from build123d import *

# Parameters (mm, degrees)
SKETCH1_W           = 25
SKETCH1_H           = 2
SKETCH2_W           = 15
SKETCH2_H           = 3.5
TAPPED_HOLE1_REACH  = 31.385
TAPPED_HOLE1_BORE_R = 1.25
CIRPATTERN1_COUNT   = 2
CIRPATTERN1_ANGLE   = 90
CHAMFER1_SIZE       = 1


with BuildPart() as part:
    # Sketch1 → Revolve1 (revolve)
    with BuildSketch(Plane.XY, mode=Mode.PRIVATE) as revolve1_sk:
        with Locations((12.5, 5)):
            Rectangle(SKETCH1_W, SKETCH1_H)
    revolve(revolve1_sk.sketch.rotate(Axis((0, 0, 0), (1, 0, 0)), 90), axis=Axis((0, 0, 0), (1, 0, 0)))

    # Sketch2 → Revolve2 (revolve)
    with BuildSketch(Plane.XY, mode=Mode.PRIVATE) as revolve2_sk:
        with Locations((7.5, 5.75)):
            Rectangle(SKETCH2_W, SKETCH2_H)
    revolve(revolve2_sk.sketch.rotate(Axis((0, 0, 0), (1, 0, 0)), 90), axis=Axis((0, 0, 0), (1, 0, 0)))

    # Tapped Hole1 bore → Tapped Hole1 (cut, up to next)
    with BuildSketch(Plane(origin=(0, 6, 0), x_dir=(1, 0, 0), z_dir=(0, 1, 0)), mode=Mode.PRIVATE) as tapped_hole1_sk1:
        with Locations((20, 0)):
            Circle(TAPPED_HOLE1_BORE_R)
    tapped_hole1_tool1 = extrude(tapped_hole1_sk1.sketch, amount=-TAPPED_HOLE1_REACH, mode=Mode.PRIVATE) & part.part
    tapped_hole1 = tapped_hole1_tool1.solids().sort_by_distance((20, 6, 0))[0]
    add(tapped_hole1, mode=Mode.SUBTRACT)

    # CirPattern1: Tapped Hole1 ×2 about axis
    cirpattern1_axis = Axis((0, 0, 0), (-1, 0, 0))
    for i in range(1, CIRPATTERN1_COUNT):
        add(tapped_hole1.rotate(cirpattern1_axis, i * CIRPATTERN1_ANGLE / (CIRPATTERN1_COUNT - 1)), mode=Mode.SUBTRACT)

    # Chamfer1
    chamfer1_edges = [part.edges().sort_by_distance(p)[0] for p in [
        (25, 0, -6),
    ]]
    chamfer(chamfer1_edges, length=CHAMFER1_SIZE)


solid = part.part
Geometry check sheet. Reference: the model listing, model coordinates, mm. A direction names the side the tool comes from. Give positions to 0.01 mm unless a question says otherwise; leave off trailing zeros. Order: outer loops, then holes, each group sorted by start corner. A loop starts at its lowest first (then second) coordinate and runs counter-clockwise, first axis right, second up. Notation, with made-up numbers: M 65.25,54.25 L 73.25,54.25 A24 ccw 73.25,83.25 Z; hole C 25.5,40 d8. An arc over 180 degrees is marked long. Use a Markdown table: item, result.
Item 1: Section check A-A (y = 0). Record the cut outline in (x, z).
Answers follow:
| item | result |
|---|---|
| outline | M 0,-7.5 L 15,-7.5 L 15,-6 L 18.75,-6 L 18.75,-4 L 0,-4 Z; M 0,4 L 25,4 L 25,5 L 24,6 L 15,6 L 15,7.5 L 0,7.5 Z; M 21.25,-6 L 24,-6 L 25,-5 L 25,-4 L 21.25,-4 Z |
Item 2: Material ranges on line 1 along Y through (x, z) = (18.5, 0); line 2 along X through (y, z) = (4.3, 0); line 3 along Y through (x, z) = (13.75, 0), recorded low to high.
Answers follow:
| item | result |
|---|---|
| line 1 | y = -6 to -4, 4 to 6 |
| line 2 | x = 0 to 18.75, 21.25 to 25 |
| line 3 | y = -7.5 to -4, 4 to 7.5 |
Item 3: Section check C-C (x = 20). Record the cut outline in (y, z), and give its area (3 significant figures).
Answers follow:
| item | result |
|---|---|
| outline | M -1.25,-5.87 L -1.25,-3.8 A4 cw long 3.8,1.25 L 5.87,1.25 A6 ccw long Z; M 1.25,-5.87 A6 ccw 5.87,-1.25 L 3.8,-1.25 A4 cw 1.25,-3.8 Z |
| area | 52.7 mm2 |
Item 4: Section check D-D (x = 2.5). Record the cut outline in (y, z).
Answers follow:
| item | result |
|---|---|
| outline | C 0,0 d15; hole C 0,0 d8 |
Item 5: Draft check along X on faces 1 (the cylindrical face through (18.75, 4.92, -0.05)), 2 (the cylindrical face through (7.605, -6.324, 4.032)), 3 (the cylindrical face through (18.75, -0.05, -4.92)), 4 (the flat face through (15, -6, -2)). Enter one of: +X half, -X half, draft (parallel to the pull), parting line (faces both ways), or undercut.
Answers follow:
| item | result |
|---|---|
| face 1 | undercut |
| face 2 | draft |
| face 3 | undercut |
| face 4 | +X half |
Item 6: Depth check by flat-ended pin: P1, Ø2, axis at x = 20, z = 0, coming from the +Y side; P2, Ø8, axis at x = 6.5, z = 5, coming from the -Y side; P3, Ø2, axis at x = 20, y = 0, coming from the +Z side. Enter the tip coordinate at first touch or a pass-through.
Answers follow:
| item | result |
|---|---|
| P1 | stops at y = -3.87 |
| P2 | stops at y = -7.43 |
| P3 | stops at z = 6 |
Item 7: Section check B-B (z = 0). Record the cut outline in (x, y), and give its area (3 significant figures).
Answers follow:
| item | result |
|---|---|
| outline | M 0,-7.5 L 15,-7.5 L 15,-6 L 24,-6 L 25,-5 L 25,-4 L 0,-4 Z; M 0,4 L 18.75,4 L 18.75,6 L 15,6 L 15,7.5 L 0,7.5 Z; M 21.25,4 L 25,4 L 25,5 L 24,6 L 21.25,6 Z |
| area | 139 mm2 |
Item 8: Tool access check on faces 5 (the cylindrical face through (12.675, 1.532, 3.695)), 6 (the cylindrical face through (19.563, -1.802, 5.723)). Record the directions out of +Z, -Z, +X, -X, +Y, -Y that give a thin tool (end or side, any length) a straight path to the whole face; none if there is none.
Answers follow:
| item | result |
|---|---|
| face 5 | +X, -X |
| face 6 | +X |
